Autodesk Inventor part; units mm, degrees
ref_plane "ANBAU_XY" through (0, 0, -285) normal (0, 0, -1) x (1, 0, 0)
ref_plane "ANBAU_YZ" through (0, 0, -285) normal (1, 0, 0) x (0, -1, 0)
ref_plane "ANBAU_ZX" through (0, 0, -285) normal (0, -1, 0) x (0, 0, -1)
sketch "Sketch_1" plane through (0, 0, 0) normal (1, 0, 0) x (0, 1, 0)
  line L0 (0, -285) -> (0, 51)
  line L1 (0, 51) -> (12, 51)
  line L2 (12, 51) -> (12.5, 50.5)
  line L3 (12.5, 50.5) -> (12.5, 40)
  line L4 (12.5, 40) -> (24.4226, 40)
  line L5 (24.4226, 40) -> (25, 39)
  line L6 (25, 39) -> (25, -251.6667)
  line L7 (25, -251.6667) -> (50, -251.6667)
  line L8 (50, -251.6667) -> (50, -285)
  line L9 (50, -285) -> (0, -285)
  line L10 (0, -285) -> (0, 51)
revolve "Revolution1" add sketch "Sketch_1" angle 360 about axis through (0, 0, -285) along (0, 0, -1)
sketch "Sketch_3" plane through (0, 0, 0) normal (0, 1, 0) x (-1, 0, 0)
  line L0 (14, 41) -> (14, 54)
  line L1 (14, 54) -> (-14, 54)
  line L2 (-14, 54) -> (-14, 41)
  line L3 (-14, 41) -> (-11, 41)
  line L4 (-11, 41) -> (-11, 51)
  line L5 (-11, 51) -> (11, 51)
  line L6 (11, 51) -> (11, 41)
  line L7 (11, 41) -> (14, 41)
extrude "Extrusion1" cut sketch "Sketch_3" along normal mid plane 50
sketch "Sketch_2" plane through (0, 0, 0) normal (1, 0, 0) x (0, 1, 0)
  line L0 (0, 51) -> (0, 91)
  line L1 (0, 91) -> (9.08, 91)
  line L2 (9.08, 91) -> (10, 90.08)
  line L3 (10, 90.08) -> (10, 54.92)
  line L4 (10, 54.92) -> (9.08, 54)
  line L5 (9.08, 54) -> (9.08, 51.6)
  arc A0 (9.08, 51.6) -> (9.68, 51) centre (9.68, 51.6) ccw
  line L6 (9.68, 51) -> (0, 51)
  line L7 (0, 51) -> (0, 91)
revolve "Revolution2" add sketch "Sketch_2" angle 360 about axis through (0, 0, 51) along (0, 0, -1)
thread "Thread1"
ref_plane "ANBAU_XY" through (0, 0, -285) normal (0, 0, -1) x (1, 0, 0)
ref_plane "ANBAU_YZ" through (0, 0, -285) normal (1, 0, 0) x (0, -1, 0)
ref_plane "ANBAU_ZX" through (0, 0, -285) normal (0, -1, 0) x (0, 0, -1)
ref_plane "NUT_XY" through (0, 0, 61) normal (0, 0, -1) x (1, 0, 0)
ref_plane "NUT_YZ" through (0, 0, 61) normal (1, 0, 0) x (0, -1, 0)
ref_plane "NUT_ZX" through (0, 0, 61) normal (0, -1, 0) x (0, 0, -1)
properties part number "ESBF-BS-100-100-20P---(KS_0)"
Check sheet for the modelled part. Datum: model origin and axes. Units: mm. A direction names the side the tool comes from. Round coordinates to 2 decimals unless told otherwise and drop trailing zeros. Write each loop counter-clockwise with the first axis right and the second up, starting at its lowest first coordinate (ties: lowest second). Pieces come first, ordered by that corner, then holes. Notation, with made-up numbers: (79.5, 57.25) - (106.5, 57.25) arc R25 ccw to (106.5, 79.25) - close; hole circle Ø9 at (65, 46). An arc over 180 degrees is marked (long way). Return JSON: item names as keys, results as strings.
Q1. Cross-section at B-B (x = 0). Record the boundary of the cut face in (y, z).
Returned:
{"outline": "(-50, -285) - (50, -285) - (50, -251.67) - (25, -251.67) - (25, 39) - (24.42, 40) - (12.5, 40) - (12.5, 50.5) - (12, 51) - (9.68, 51) arc R0.6 cw to (9.08, 51.6) - (9.08, 54) - (10, 54.92) - (10, 90.08) - (9.08, 91) - (-9.08, 91) - (-10, 90.08) - (-10, 54.92) - (-9.08, 54) - (-9.08, 51.6) arc R0.6 cw to (-9.68, 51) - (-12, 51) - (-12.5, 50.5) - (-12.5, 40) - (-24.42, 40) - (-25, 39) - (-25, -251.67) - (-50, -251.67) - close"}
Q2. Cross-section at C-C (z = 29.5). Record the boundary of the cut face in (x, y).
Returned:
{"outline": "circle Ø50 at (0, 0)"}
Q3. Depth check by flat-ended pin: P1, Ø3, axis at y = 2, z = 47, coming from the -X side; P2, Ø12, axis at x = -14.5, y = -7, coming from the +Z side; P3, Ø1.5, axis at y = -17, z = -54, coming from the +X side. Enter the tip coordinate at first touch or a pass-through.
Returned:
{"P1": "stops at x = -11", "P2": "stops at z = 51", "P3": "stops at x = 19"}
Q4. Draft check along Z on faces 5 (the flat face through (-11, 0, 46)), 6 (the cylindrical face through (-5.525, -7.206, 52.783)), 7 (the conical face through (0.2, -12.14, 50.86)). Enter one of: released by +Z, released by -Z, zero draft, split by the parting line, or undercut.
Returned:
{"face 5": "zero draft", "face 6": "undercut", "face 7": "released by +Z"}
Q5. Cross-section at D-D (x = -38). Record the boundary of the cut face in (y, z), then the cut area to 3 significant figures.
Returned:
{"outline": "(-32.5, -285) - (32.5, -285) - (32.5, -251.67) - (-32.5, -251.67) - close", "area": "2,170 mm²"}
Q6. Access from +Z, -Z, +X, -X, +Y, -Y to the whole of each face (thin tool, end or side, straight path). Record for faces 1 (the cylindrical face through (7.509, 23.846, -108.368)), 2 (the conical face through (-0.2, 12.14, 50.86)), 3 (the flat face through (10, 0, 51)), 4 (the flat face through (11, 0, 46)).
Returned:
{"face 1": "+Z", "face 2": "+Z, +Y", "face 3": "none", "face 4": "+Z, +X, +Y, -Y"}
Q7. Scan lines: L1, parallel to X at y = -5, z = -121; L2, parallel to Z at x = -23, y = -36; L3, parallel to Z at x = 11, y = -17. Record each from-to range of solid material in increasing order. Write a range as from..to.
Returned:
{"L1": "x = -24.49..24.49", "L2": "z = -285..-251.67", "L3": "z = -285..40"}
